Design review of the part built by this model. Coordinates are the model's own, in mm. Face numbers are marked on the shaded views. A direction names the side the tool comes from. Give positions to 0.01 mm unless a question says otherwise; leave off trailing zeros. Write each loop counter-clockwise with the first axis right and the second up, starting at its lowest first coordinate (ties: lowest second). Pieces come first, ordered by that corner, then holes. Notation, with made-up numbers: (-7.75, 25) -> (12.25, 25) arc R25 cw to (12.25, 61) -> close; hole circle Ø4 at (53, 49.5). An arc over 180 degrees is marked (long way). Use CSV: the item, a comma, the result in double quotes.
```python
from build123d import *

# Parameters (mm, degrees)
F0_W     = 31.75
F0_H     = 19.05
F1_DEPTH = 9.525
F3_D     = 5.1054
F5_D     = 4.0386
F5_DEPTH = 15.875
F5_TIP   = 1.213317848
F6_SIZE  = 6.35


with BuildPart() as f1:
    # F0 (on Front) → F1 (new body)
    with BuildSketch(Plane.XZ):
        Rectangle(F0_W, F0_H)
    extrude(amount=F1_DEPTH)

    # F3 (through all)
    with Locations(Plane.XZ.offset(9.525)):
        with Locations((7.9502, 0)):
            Hole(F3_D / 2)

    # F5
    with Locations(Plane.XY.offset(9.525)):
        with Locations((-9.525, -4.7625), (0, -4.7625)):
            Hole(F5_D / 2, depth=F5_DEPTH)
            with Locations((0, 0, -(F5_DEPTH + F5_TIP / 2))):  # 118° drill point
                Cone(0, F5_D / 2, F5_TIP, mode=Mode.SUBTRACT)

    # F6
    f6_edges = [f1.edges().sort_by_distance(p)[0] for p in [
        (-15.875, -4.7625, -9.525),
        (15.875, -4.7625, -9.525),
    ]]
    chamfer(f6_edges, length=F6_SIZE)


solid = f1.part
```
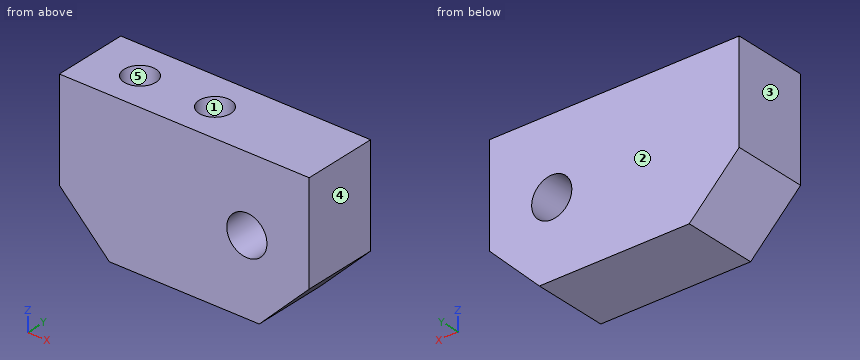
(1) Take a section at C-C (x = 8). Write out the cut boundary in (y, z) (3 decimals), then the cut area to 3 significant figures.
Established:
outline,"(-9.525, -9.525) -> (0, -9.525) -> (0, -2.552) -> (-9.525, -2.552) -> close; (-9.525, 2.552) -> (0, 2.552) -> (0, 9.525) -> (-9.525, 9.525) -> close"
area,"133 mm2"
(2) Tool access review of the marked faces 4 and 5: name each direction out of +Z, -Z, +X, -X, +Y, -Y from which nothing blocks a thin tool from reaching the whole face with its end or side.
Established:
face 4,"+Z, -Z, +X, +Y, -Y"
face 5,"+Z"
(3) Take a section at A-A (z = 0). Write out the cut boundary in (x, y) (1 decimal).
Established:
outline,"(-15.9, -9.5) -> (5.4, -9.5) -> (5.4, 0) -> (-15.9, 0) -> close; (10.5, -9.5) -> (15.9, -9.5) -> (15.9, 0) -> (10.5, 0) -> close; hole circle Ø4 at (-9.5, -4.8); hole circle Ø4 at (0, -4.8)"
(4) Take a section at B-B (y = -0.75). Write out the cut boundary in (x, z) (1 decimal).
Established:
outline,"(-15.9, -3.2) -> (-9.5, -9.5) -> (9.5, -9.5) -> (15.9, -3.2) -> (15.9, 9.5) -> (-15.9, 9.5) -> close; hole circle Ø5.1 at (8, 0)"
(5) For line 1 along Y through (x, z) = (0, 1.75) (3 decimals); line 2 along X through (y, z) = (-6.25, 5.25) (3 decimals); line 3 along X through (y, z) = (-5, 2) (3 decimals), list the stretches that pass through material, from the lowest coordinate up. Write a range as [from, to].
Established:
line 1,"y = [-9.525, -6.782], [-2.743, 0]"
line 2,"x = [-15.875, -10.891], [-8.159, -1.366], [1.366, 15.875]"
line 3,"x = [-15.875, -11.53], [-7.52, -2.005], [2.005, 6.364], [9.536, 15.875]"
(6) Mouldability with a two-part tool opening along X and no side actions: class the marked faces 1, 2 and 3 as +X half, -X half, draft (parallel to the pull), parting line (faces both ways), or undercut.
Established:
face 1,"undercut"
face 2,"draft"
face 3,"-X half"
(7) Take a section at D-D (z = -3.75). Write out the cut boundary in (x, y) (1 decimal), then the cut area to 3 significant figures.
Established:
outline,"(-15.3, -9.5) -> (15.3, -9.5) -> (15.3, 0) -> (-15.3, 0) -> close; hole circle Ø4 at (-9.5, -4.8); hole circle Ø4 at (0, -4.8)"
area,"266 mm2"
